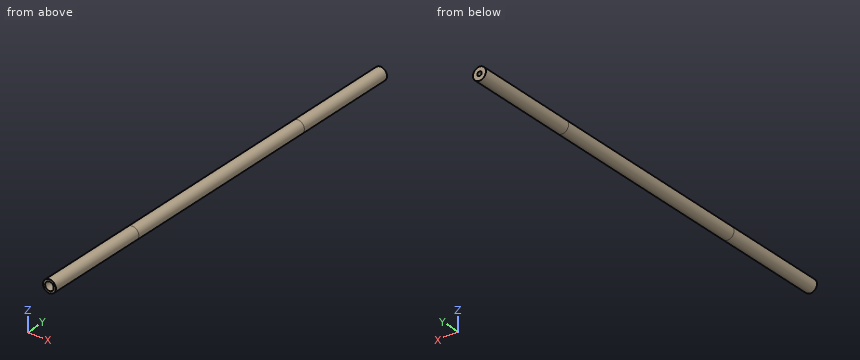
from build123d import *

# Parameters (mm, degrees)
SKETCH1_R                 = 1.5
SKETCH1_R_2               = 0.5
F_2_0MM_DOWEL_HOLE1_D     = 2
F_2_0MM_DOWEL_HOLE1_DEPTH = 7.5
F_2_0MM_DOWEL_HOLE1_TIP   = 0.600860619


with BuildPart() as part:
    # Sweep1: sweep along a path in Sketch2
    with BuildLine(Plane.XY) as sweep1_path:
        Line((0, 0), (0, 25))
        ThreePointArc((0, 25), (-0.015624988, 50.000019531), (-0.062499927, 75))
        Line((-0.062499927, 75), (-0.124999951, 100))
    # Sketch1 → Sweep1 (sweep)
    with BuildSketch(Plane(origin=(0, 0, 0), x_dir=(1, 0, 0), z_dir=(0, 1, 0))):
        Circle(SKETCH1_R)
        Circle(SKETCH1_R_2, mode=Mode.SUBTRACT)
    sweep(path=sweep1_path.line)

    # Ø2.0mm Dowel Hole1
    with Locations(Plane(origin=(0, 0, 0), x_dir=(-1, 0, 0), z_dir=(0, -1, 0))):
        with Locations((0, 0)):
            Hole(F_2_0MM_DOWEL_HOLE1_D / 2, depth=F_2_0MM_DOWEL_HOLE1_DEPTH)
            with Locations((0, 0, -(F_2_0MM_DOWEL_HOLE1_DEPTH + F_2_0MM_DOWEL_HOLE1_TIP / 2))):  # 118° drill point
                Cone(0, F_2_0MM_DOWEL_HOLE1_D / 2, F_2_0MM_DOWEL_HOLE1_TIP, mode=Mode.SUBTRACT)


solid = part.part
Source: CAD feature listing. Evaluate the final solid. Frame: model axes, mm. Give positions to 0.01 mm unless a question says otherwise; leave off trailing zeros. Write each loop counter-clockwise with the first axis right and the second up, starting at its lowest first coordinate (ties: lowest second). Pieces come first, ordered by that corner, then holes. Notation, with made-up numbers: M 29.5,49 L 76.5,49 A27 ccw 76.5,76 Z; hole C 8.5,15.5 d6. An arc over 180 degrees is marked long. Return JSON: item names as keys, results as strings. Group by question number.
1) Material intervals for line 1 along Z through (x, y) = (0, 19.25); line 2 along Z through (x, y) = (0, 3.25); line 3 along X through (y, z) = (8.5, 0.1), sorted ascending. Write a range as [from, to].
2) Cut plane A-A, the plane z = 0. Output: boundary loops of the cut face in (x, y) (1 decimal).
3) Pin query (flat end, axial travel): P1, Ø1.5, axis at y = 70, z = 0.5, coming from the -X side; P2, Ø1, axis at x = -1, y = 67.5, coming from the -Z side. Return the tip coordinate at first contact, or that it passes through.
Recorded:
{
 "1": {"line 1": "z = [-1.5, -0.5], [0.5, 1.5]", "line 2": "z = [-1.5, -1], [1, 1.5]", "line 3": "x = [-1.5, -0.49], [0.49, 1.5]"},
 "2": {"outline": "M -1.6,75 A19998.6 cw -1.5,25 L -1.5,0 L -1,0 L -1,7.5 L -0.5,7.8 L -0.5,25 A19999.6 ccw -0.6,75 L -0.6,100 L -1.6,100 Z; M 0.4,75 A20000.6 cw 0.5,25 L 0.5,7.8 L 1,7.5 L 1,0 L 1.5,0 L 1.5,25 A20001.6 ccw 1.4,75 L 1.4,100 L 0.4,100 Z"},
 "3": {"P1": "stops at x = -1.55", "P2": "stops at z = -1.43"}
}
